Work out the finished part from the listing and answer in its coordinate system (mm). Give positions to 0.01 mm unless a question says otherwise; leave off trailing zeros. Order: outer loops, then holes, each group sorted by start corner. A loop starts at its lowest first (then second) coordinate and runs counter-clockwise, first axis right, second up. Notation, with made-up numbers: (65.25, 23.25) - (72.25, 23.25) arc R32 ccw to (72.25, 59.25) - close; hole circle Ø11 at (45.25, -36.5). An arc over 180 degrees is marked (long way). Return JSON: item names as keys, results as strings. Group by question number.
from build123d import *

# Parameters (mm, degrees)
F0_W     = 19.05
F0_H     = 19.05
F1_DEPTH = 19.05
F2_R     = 6.35
F3_DEPTH = 25.4


with BuildPart() as f1:
    # F0 (on Front) → F1 (new body)
    with BuildSketch(Plane.XZ):
        with Locations((9.525, -9.525)):
            Rectangle(F0_W, F0_H)
    extrude(amount=F1_DEPTH)

    # F2 (on face) → F3 (cut)
    with BuildSketch(Plane.XY):
        with Locations((9.525, -9.525)):
            Circle(F2_R)
    extrude(amount=-F3_DEPTH, mode=Mode.SUBTRACT)


solid = f1.part
1. Consider probe 1 along Y at (x, z) = (9.75, -9.5); probe 2 along X at (y, z) = (-14.25, -11.25); probe 3 along X at (y, z) = (-11.5, -5.75). Determine where each line is inside the solid, lowest interval first. Write a range as from..to.
2. The part is cut by section A-A (x = 6). Give the vertices of the cut face in (y, z).
3. This flat-tipped pin is pushed along its axis until it touches: pin 1 (7.5 mm diameter, centred on x = 9.525, y = -9.525, fed in from -Z) (3 decimals). Where does it stop, or does it pass through?
4. The part is cut by section C-C (z = -6.25). Give the vertices of the cut face in (x, y) (3 decimals), and give its area (3 significant figures).
5. The part is cut by section B-B (y = -7.5). Give the vertices of the cut face in (x, z).
6. Determine the mould class of faces 1 (the flat face through (19.05, -9, -10)), 2 (the flat face through (0, -9, -10)), 3 (the cylindrical face through (15.582, -7.618, -9.392)) for opening direction X: released by +X, released by -X, zero draft, split by the parting line, or undercut.
Answers:
{
 "1": {"probe 1": "y = -19.05..-15.87, -3.18..0", "probe 2": "x = 0..5.28, 13.77..19.05", "probe 3": "x = 0..3.49, 15.56..19.05"},
 "2": {"outline": "(-19.05, -19.05) - (-14.81, -19.05) - (-14.81, 0) - (-19.05, 0) - close; (-4.24, -19.05) - (0, -19.05) - (0, 0) - (-4.24, 0) - close"},
 "3": {"pin 1": "passes through"},
 "4": {"outline": "(0, -19.05) - (19.05, -19.05) - (19.05, 0) - (0, 0) - close; hole circle Ø12.7 at (9.525, -9.525)", "area": "236 mm^2"},
 "5": {"outline": "(0, -19.05) - (3.51, -19.05) - (3.51, 0) - (0, 0) - close; (15.54, -19.05) - (19.05, -19.05) - (19.05, 0) - (15.54, 0) - close"},
 "6": {"face 1": "released by +X", "face 2": "released by -X", "face 3": "undercut"}
}
